```python
from build123d import *

# Parameters (mm, degrees)
SKETCH2_W          = 12.190003068
SKETCH2_H          = 1
CUT_EXTRUDE1_DEPTH = 1


with BuildPart() as part:
    # Sketch1 → Revolve1 (revolve)
    with BuildSketch(Plane.XY, mode=Mode.PRIVATE) as revolve1_sk:
        with BuildLine():
            Line((0, 0), (14.25, 0))
            Line((14.25, 0), (14.25, 2))
            Line((14.25, 2), (2.25, 2))
            Line((2.25, 2), (2.25, 3.875))
            Line((2.25, 3.875), (1.5, 3.875))
            ThreePointArc((1.5, 3.875), (0.439339828, 3.435660172), (0, 2.375))
            Line((0, 2.375), (0, 0))
        make_face()
    revolve(revolve1_sk.sketch.rotate(Axis((0, 0, 0), (-1, 0, 0)), 90), axis=Axis((0, 0, 0), (-1, 0, 0)))

    # Sketch2 → Cut-Extrude1 (cut)
    with BuildSketch(Plane.ZY):
        Rectangle(SKETCH2_W, SKETCH2_H)
    extrude(amount=-CUT_EXTRUDE1_DEPTH, mode=Mode.SUBTRACT)


solid = part.part
```
Check sheet for the modelled part. Datum: model origin and axes. Units: mm. A direction names the side the tool comes from. Give positions to 0.01 mm unless a question says otherwise; leave off trailing zeros. Order: outer loops, then holes, each group sorted by start corner. A loop starts at its lowest first (then second) coordinate and runs counter-clockwise, first axis right, second up. Notation, with made-up numbers: M 58.25,-28.75 L 88.25,-28.75 A6 ccw 88.25,-22.75 Z; hole C -15,62.25 d8. An arc over 180 degrees is marked long. Answer in a Markdown table with one row per item.
1) Cross-section at A-A, the plane z = 0. Enter the section's corners in (x, y) (3 decimals), plus the area to 3 significant figures.
Filled sheet:
| item | result |
|---|---|
| outline | M 0,-2.375 A1.5 ccw 1.5,-3.875 L 2.25,-3.875 L 2.25,-2 L 14.25,-2 L 14.25,2 L 2.25,2 L 2.25,3.875 L 1.5,3.875 A1.5 ccw 0,2.375 L 0,0.5 L 1,0.5 L 1,-0.5 L 0,-0.5 Z |
| area | 63.5 mm2 |
2) Thickness scan on L1, parallel to X at y = 1.25, z = -2; L2, parallel to Z at x = 7, y = -1; L3, parallel to Z at x = 1.5, y = -3.25. Record the ranges inside material, lowest first. Write a range as [from, to].
Filled sheet:
| item | result |
|---|---|
| L1 | x = [0, 2.25] |
| L2 | z = [-1.73, 1.73] |
| L3 | z = [-2.11, 2.11] |
3) Access from +Z, -Z, +X, -X, +Y, -Y to the whole of each face (thin tool, end or side, straight path). Record for faces 1 (the flat face through (0, 1, 0)), 2 (the flat face through (0.5, -0.5, -0.1)), 3 (the flat face through (2.25, 2, 2)).
Filled sheet:
| item | result |
|---|---|
| face 1 | +Z, -Z, -X, +Y, -Y |
| face 2 | +Z, -Z, -X |
| face 3 | +X |
4) Gauge pin test, flat ends, axial feed: P1, Ø4, axis at x = 5.5, z = 2, coming from the +Y side; P2, Ø4, axis at x = 9.5, z = 1, coming from the -Y side; P3, Ø1, axis at x = 4.5, z = 1, coming from the -Y side. Record the tip position at first contact, or that the pin passes through.
Filled sheet:
| item | result |
|---|---|
| P1 | stops at y = 2 |
| P2 | stops at y = -2 |
| P3 | stops at y = -1.94 |
5) Cross-section at B-B, the plane x = 8.25. Enter the section's corners in (y, z).
Filled sheet:
| item | result |
|---|---|
| outline | C 0,0 d4 |
